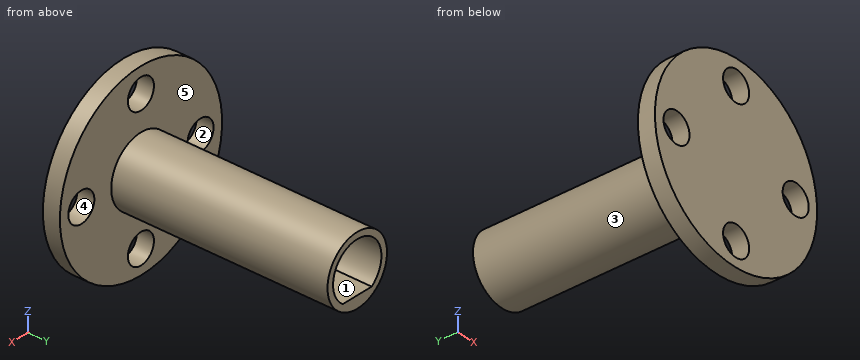
from build123d import *

# Parameters (mm, degrees)
SKETCH3_R           = 4
BOSS_EXTRUDE1_DEPTH = 27.4
SKETCH3_17_R        = 10.9
SKETCH3_17_R_2      = 1.75
BOSS_EXTRUDE2_DEPTH = 2


with BuildPart() as part:
    # Sketch3 → Boss-Extrude1 (new body)
    with BuildSketch(Plane(origin=(0, 0, 0), x_dir=(1, 0, 0), z_dir=(0, 1, 0))):
        with Locations(Location((0, 0, 0), (0, 0, 90))):
            Circle(SKETCH3_R)
        with BuildLine():
            Line((-1.942645776, 2.605499451), (1.942645776, 2.605499451))
            ThreePointArc((1.942645776, 2.605499451), (0, -3.25), (-1.942645776, 2.605499451))
        make_face(mode=Mode.SUBTRACT)
    extrude(amount=BOSS_EXTRUDE1_DEPTH)

    # Sketch3_17 → Boss-Extrude2 (add)
    with BuildSketch(Plane(origin=(0, 0, 0), x_dir=(1, 0, 0), z_dir=(0, 1, 0))):
        with Locations(Location((0, 0, 0), (0, 0, 270))):
            Circle(SKETCH3_17_R)
        with Locations(Location((0.009034474, 8.115584077, 0), (0, 0, 270))):
            Circle(SKETCH3_17_R_2, mode=Mode.SUBTRACT)
        with Locations(Location((8.017679827, 0.053335715, 0), (0, 0, 270))):
            Circle(SKETCH3_17_R_2, mode=Mode.SUBTRACT)
        with Locations(Location((0.009179949, -8.009057152, 0), (0, 0, 270))):
            Circle(SKETCH3_17_R_2, mode=Mode.SUBTRACT)
        with Locations(Location((-7.999465404, 0.05319121, 0), (0, 0, 270))):
            Circle(SKETCH3_17_R_2, mode=Mode.SUBTRACT)
    extrude(amount=BOSS_EXTRUDE2_DEPTH)


solid = part.part
Design review of the part built by this model. Coordinates are the model's own, in mm. Face numbers are marked on the shaded views. A direction names the side the tool comes from. Coordinates: 2 decimals unless noted, no trailing zeros. Order: outer loops, then holes, each group sorted by start corner. A loop starts at its lowest first (then second) coordinate and runs counter-clockwise, first axis right, second up. Notation, with made-up numbers: (-8, -24) - (2, -24) arc R19 ccw to (2, -10) - close; hole circle Ø10 at (-20.5, 81.25). An arc over 180 degrees is marked (long way). Put each result on its own line as item: value.
1) Take a section at A-A, the plane z = 7.75. Give the boundary of the cut face in (x, y), and give its area (3 significant figures).
Response values:
outline: (-7.66, 0) - (-1.72, 0) - (-1.72, 2) - (-7.66, 2) - close; (1.74, 0) - (7.66, 0) - (7.66, 2) - (1.74, 2) - close
area: 23.7 mm²
2) The part is to be moulded in two halves that separate along X. For the marked faces 3, 4 and 5, say which applies: released by +X, released by -X, zero draft, split by the parting line, or undercut.
Response values:
face 3: split by the parting line
face 4: undercut
face 5: zero draft
3) Tool access review of the marked faces 1 and 2: name each direction out of +Z, -Z, +X, -X, +Y, -Y from which nothing blocks a thin tool from reaching the whole face with its end or side.
Response values:
face 1: +Y
face 2: +Y, -Y
4) Wall thickness on L1, parallel to Y at x = 4.5, z = 0; L2, parallel to Z at x = -2.5, y = 25.5; L3, parallel to X at y = 25, z = 1.75: over which ranges is each line inside the solid? List them lowest first. Write a range as from..to.
Response values:
L1: y = 0..2
L2: z = -3.12..-2.08, 2.08..3.12
L3: x = -3.6..-2.74, 2.74..3.6
5) Take a section at C-C, the plane z = 0. Give the boundary of the cut face in (x, y).
Response values:
outline: (-10.9, 0) - (-9.75, 0) - (-9.75, 2) - (-10.9, 2) - close; (-6.25, 0) - (6.27, 0) - (6.27, 2) - (4, 2) - (4, 27.4) - (3.25, 27.4) - (3.25, 2) - (-3.25, 2) - (-3.25, 27.4) - (-4, 27.4) - (-4, 2) - (-6.25, 2) - close; (9.77, 0) - (10.9, 0) - (10.9, 2) - (9.77, 2) - close
6) Take a section at B-B, the plane x = -7.25. Give the boundary of the cut face in (y, z), and give its area (3 significant figures).
Response values:
outline: (0, -8.14) - (2, -8.14) - (2, -1.63) - (0, -1.63) - close; (0, 1.53) - (2, 1.53) - (2, 8.14) - (0, 8.14) - close
area: 26.2 mm²
7) Insertion check: P1, Ø1.2, axis at x = 1, y = 11, coming from the +Z side; P2, Ø2, axis at x = -8.5, z = 7.5, coming from the +Y side; P3, Ø5, axis at x = -3.5, y = 10.5, coming from the -Z side. Each pin has a flat end and moves straight along its axis. Give the tip position at first contact, or say it passes through.
Response values:
P1: stops at z = 3.98
P2: stops at y = 2
P3: stops at z = -3.87
8) Take a section at D-D, the plane y = 3. Give the boundary of the cut face in (x, z), and give its area (3 significant figures).
Response values:
outline: circle Ø8 at (0, 0); hole (-1.94, -2.61) - (1.94, -2.61) arc R3.25 ccw (long way) to start
area: 18.8 mm²
